Can you work these out from the model? Positions are in its coordinate system, mm. A direction names the side the tool comes from. Coordinates: 2 decimals unless noted, no trailing zeros. Loops run counter-clockwise (first coordinate to the right, second up) from the corner with the lowest first, then second, coordinate; pieces in that order, holes last. Notation, with made-up numbers: M 87.25,65 L 137.25,65 A28 cw 137.25,98 Z; hole C 22.25,35.25 d3. An arc over 180 degrees is marked long. Answer as a JSON object with one key per item and string values. Group by question number.
Item 1: Suppose I cut it at A-A (z = 15.5). Write out the boundary of the cut face in (x, y).
Item 2: If I drill on line 1 (Y direction, x = -52, z = 13.75); line 2 (Z direction, x = -55.75, y = 3.5); line 3 (X direction, y = -4.5, z = 14.5), over which ranges is the centre line in solid material (lowest first)?
Item 3: I'm going to push flat-ended pins straight in: pin 1 Ø4 at (x, y) = (-54.5, -3.5) entering from -Z; pin 2 Ø4 at (y, z) = (-2.5, 15) entering from -X; pin 3 Ø3 at (x, y) = (-56, 6) entering from +Z. Where does each tip first touch, or does it pass through?
Item 4: Suppose I cut it at B-B (x = -53.25). Write out the boundary of the cut face in (y, z).
Item 5: Which directions (+Z, -Z, +X, -X, +Y, -Y) give clear straight access to the entire face, cutting with the end or side of a thin tool? Please do faces 1 (the flat face through (-56.158, -3, 14)), 2 (the flat face through (-52.729, 6, 14)), 3 (the flat face through (-54, -3, 12.701)), 4 (the flat face through (-54, 6, 12.701)), 5 (the flat face through (-56.158, 6, 14)).
Item 6: Suppose I cut it at C-C (y = 6). Write out the boundary of the cut face in (x, z).
Item 7: Suppose I cut it at D-D (x = -51.5). Write out the boundary of the cut face in (y, z).
Item 8: We'd pull the mould along Y, two halves only. Please class faces 6 (the flat face through (-58.531, 1, 15)), 7 (the flat face through (-54, 10.668, 14)), 8 (the flat face through (-54, -5.842, 14)): +Y half, -Y half, draft (parallel to the pull), parting line (faces both ways), or undercut.
```python
from build123d import *

# Parameters (mm, degrees)
F0_W          = 3.429
F0_H          = 3.429
F1_DEPTH      = 5.842
F1_DEPTH_BACK = 10.668
F0_W_2        = 8.001
F0_H_2        = 8.001
F2_DEPTH      = 1.778


with BuildPart() as f1:
    # F0 (on Front) → F1 (new body, two sides)
    with BuildSketch(Plane.XZ) as f1_sk:
        with Locations((-54.44314, 14.415071)):
            Rectangle(F0_W, F0_H)
    extrude(amount=F1_DEPTH)
    extrude(f1_sk.sketch, amount=-F1_DEPTH_BACK)

    # F0 (on Front) → F2 (join)
    with BuildSketch(Plane.XZ):
        with Locations((-54.53074, 14.837216)):
            Rectangle(F0_W_2, F0_H_2)
        with Locations((-54.44314, 14.415071)):
            Rectangle(F0_W, F0_H, mode=Mode.SUBTRACT)
    extrude(amount=-F2_DEPTH)


solid = f1.part
```
From the geometry:
{
 "1": {"outline": "M -58.53,0 L -56.16,0 L -56.16,-5.84 L -52.73,-5.84 L -52.73,0 L -50.53,0 L -50.53,1.78 L -52.73,1.78 L -52.73,10.67 L -56.16,10.67 L -56.16,1.78 L -58.53,1.78 Z"},
 "2": {"line 1": "0 to 1.78", "line 2": "12.7 to 16.13", "line 3": "-56.16 to -52.73"},
 "3": {"pin 1": "z = 12.7", "pin 2": "x = -56.16", "pin 3": "z = 16.13"},
 "4": {"outline": "M -5.84,12.7 L 0,12.7 L 0,10.84 L 1.78,10.84 L 1.78,12.7 L 10.67,12.7 L 10.67,16.13 L 1.78,16.13 L 1.78,18.84 L 0,18.84 L 0,16.13 L -5.84,16.13 Z"},
 "5": {"face 1": "+Z, -Z, -X, -Y", "face 2": "+Z, -Z, +X, +Y", "face 3": "-Z, +X, -X, -Y", "face 4": "-Z, +X, -X, +Y", "face 5": "+Z, -Z, -X, +Y"},
 "6": {"outline": "M -56.16,12.7 L -52.73,12.7 L -52.73,16.13 L -56.16,16.13 Z"},
 "7": {"outline": "M 0,10.84 L 1.78,10.84 L 1.78,18.84 L 0,18.84 Z"},
 "8": {"face 6": "draft", "face 7": "+Y half", "face 8": "-Y half"}
}
